Design review of the part shown in the three views and the two pictorial views. Dimensions are in mm from the part's minimum x, y and z. Coordinates: 2 decimals unless noted, no trailing zeros. Loops run counter-clockwise (first coordinate to the right, second up) from the corner with the lowest first, then second, coordinate; pieces in that order, holes last. Notation, with made-up numbers: (-7, -5) - (2, -5) arc R31 ccw to (2, 32) - close; hole circle Ø6 at (7, 73.25). An arc over 180 degrees is marked (long way). One line per question, with ' | ' between items.
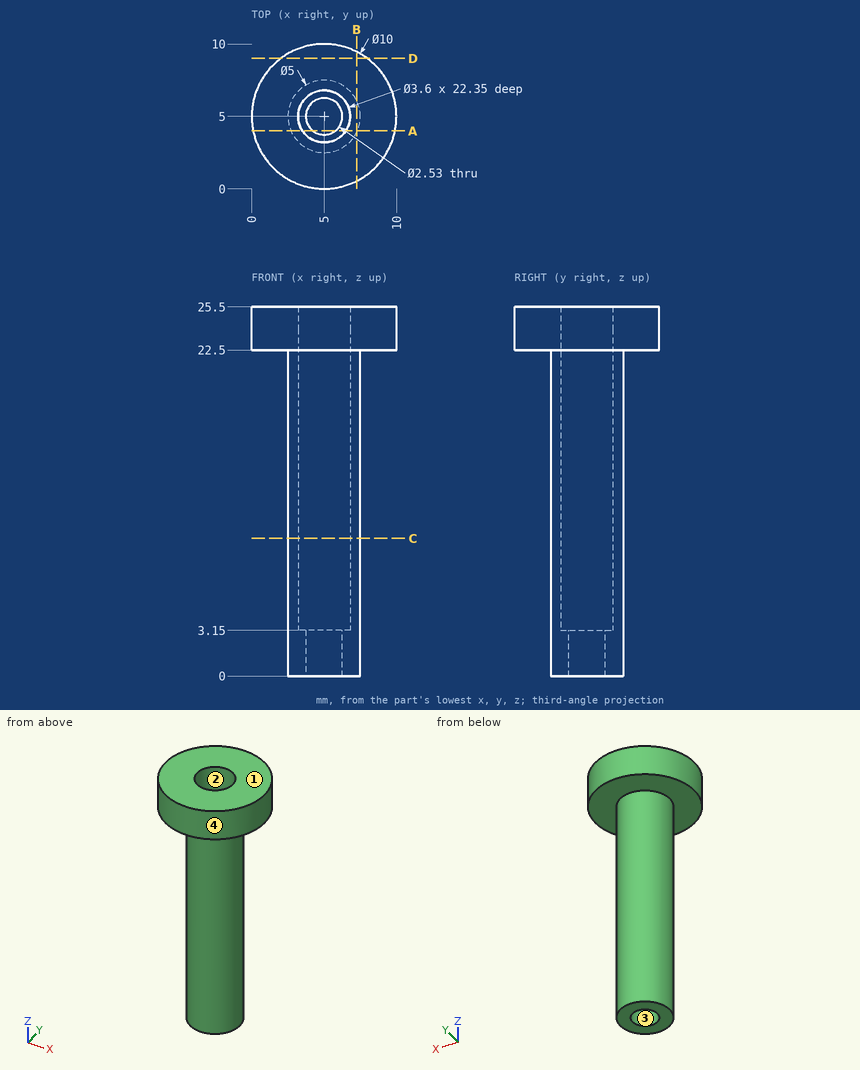
Q1. Take a section at C-C (z = 9.5). Give the boundary of the cut face in (x, y).
Returned:
outline: circle Ø5 at (5, 5); hole circle Ø3.6 at (5, 5)
Q2. To check wall thickness, follow line 1 along X through (y, z) = (5, 1.3) (3 decimals); line 2 along X through (y, z) = (5, 9). State the ranges of each line that lie inside material, in increasing order.
Returned:
line 1: x = 2.5 to 3.735, 6.265 to 7.5 | line 2: x = 2.5 to 3.2, 6.8 to 7.5
Q3. Take a section at A-A (y = 4). Give the boundary of the cut face in (x, z), plus the area to 3 significant figures.
Returned:
outline: (0.1, 22.5) - (2.71, 22.5) - (2.71, 0) - (4.23, 0) - (4.23, 3.15) - (3.5, 3.15) - (3.5, 25.5) - (0.1, 25.5) - close; (5.77, 0) - (7.29, 0) - (7.29, 22.5) - (9.9, 22.5) - (9.9, 25.5) - (6.5, 25.5) - (6.5, 3.15) - (5.77, 3.15) - close | area: 60.7 mm²
Q4. Take a section at B-B (x = 7.25). Give the boundary of the cut face in (y, z), plus the area to 3 significant figures.
Returned:
outline: (0.53, 22.5) - (3.91, 22.5) - (3.91, 0) - (6.09, 0) - (6.09, 22.5) - (9.47, 22.5) - (9.47, 25.5) - (0.53, 25.5) - close | area: 75.8 mm²
Q5. For pin 1 (2 mm diameter, centred on x = 5.5, y = 5.5, fed in from +Z); pin 2 (1.5 mm diameter, centred on x = 5, y = 5, fed in from -Z); pin 3 (6 mm diameter, centred on y = 3.5, z = 11.5, fed in from +X); pin 4 (1 mm diameter, centred on y = 5.5, z = 18.5, fed in from -X), all flat-tipped, find the tip position at first contact; note any pin that passes through.
Returned:
pin 1: stops at z = 3.15 | pin 2: passes through | pin 3: stops at x = 7.5 | pin 4: stops at x = 2.5
Q6. Draft analysis for pull direction X (two halves, no side actions). For the marked faces 1, 2, 3 and 4, state which applies: +X half, -X half, draft (parallel to the pull), parting line (faces both ways), or undercut.
Returned:
face 1: draft | face 2: undercut | face 3: undercut | face 4: parting line
Q7. Take a section at D-D (y = 9). Give the boundary of the cut face in (x, z), plus the area to 3 significant figures.
Returned:
outline: (2, 22.5) - (8, 22.5) - (8, 25.5) - (2, 25.5) - close | area: 18.0 mm²
